Could you check a few things on this model? Use its own coordinates, in mm. Face numbers are marked on the shaded views. A direction names the side the tool comes from. Coordinates: 2 decimals unless noted, no trailing zeros. Loops run counter-clockwise (first coordinate to the right, second up) from the corner with the lowest first, then second, coordinate; pieces in that order, holes last.
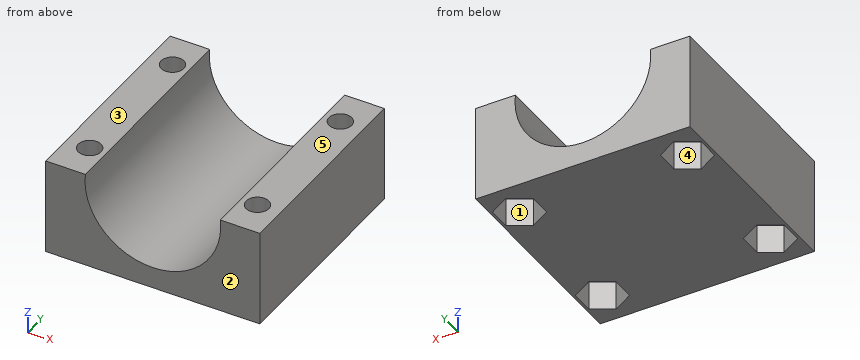
from build123d import *

# Parameters (mm, degrees)
F0_W     = 30
F0_H     = 30
F0_R     = 1.6
F1_DEPTH = 13.5
F2_R     = 9.5
F3_DEPTH = 30.001
F5_DEPTH = 4


with BuildPart() as f1:
    # F0 (on Top) → F1 (new body)
    with BuildSketch(Plane.XY):
        Rectangle(F0_W, F0_H)
        with Locations((-11.75, -10)):
            Circle(F0_R, mode=Mode.SUBTRACT)
        with Locations((11.75, -10)):
            Circle(F0_R, mode=Mode.SUBTRACT)
        with Locations((-11.75, 10)):
            Circle(F0_R, mode=Mode.SUBTRACT)
        with Locations((11.75, 10)):
            Circle(F0_R, mode=Mode.SUBTRACT)
    extrude(amount=F1_DEPTH)

    # F2 (on face) → F3 (cut, through all)
    with BuildSketch(Plane.XZ.offset(15)):
        with Locations((0, 12.5)):
            Circle(F2_R)
    extrude(amount=-F3_DEPTH, mode=Mode.SUBTRACT)

    # F4 (on face) → F5 (cut)
    with BuildSketch(Plane(origin=(0, 0, 0), x_dir=(1, 0, 0), z_dir=(0, 0, -1))):
        Polygon((-8.9, 8.354552), (-8.9, 11.645448), (-11.75, 13.290897), (-14.6, 11.645448), (-14.6, 8.354552), (-11.75, 6.709103), align=None)
        Polygon((14.6, 11.645448), (11.75, 13.290897), (8.9, 11.645448), (8.9, 8.354552), (11.75, 6.709103), (14.6, 8.354552), align=None)
        Polygon((14.6, -11.645448), (14.6, -8.354552), (11.75, -6.709103), (8.9, -8.354552), (8.9, -11.645448), (11.75, -13.290897), align=None)
        Polygon((-11.75, -13.290897), (-8.9, -11.645448), (-8.9, -8.354552), (-11.75, -6.709103), (-14.6, -8.354552), (-14.6, -11.645448), align=None)
    extrude(amount=-F5_DEPTH, mode=Mode.SUBTRACT)


solid = f1.part
1) Imagine slicing it at B-B on y = 10. List the corners of the cut face in (x, z) for me.
2) Imagine slicing it at A-A on z = 12.5. List the corners of the cut face in (x, y) for me.
3) We'd pull the mould along Y, two halves only. Please class the marked faces 1, 2 and 3: released by +Y, released by -Y, zero draft, split by the parting line, or undercut.
4) Will these pins go through, and if not, where does the flat tip stop? pin 1 (1.7 mm diameter, centred on x = -12, y = 10.5, fed in from -Z); pin 2 (5 mm diameter, centred on x = 11.75, y = 10, fed in from -Z).
5) Imagine slicing it at D-D on z = 6.5. List the corners of the cut face in (x, y) for me.
6) If I drill on L1, parallel to Y at x = -11.75, z = 6; L2, parallel to X at y = 6, z = 12.5; L3, parallel to X at y = 10, z = 9, over which ranges is the centre line in solid material (lowest first)?
7) For the marked faces 4 and 5, which set-ups out of +Z, -Z, +X, -X, +Y, -Y let a thin tool reach every point of the face, with its end or its side?
8) Imagine slicing it at C-C on y = 3.5. List the corners of the cut face in (x, z) for me.
Solved:
1. outline: (-15, 0) - (-14.6, 0) - (-14.6, 4) - (-13.35, 4) - (-13.35, 13.5) - (-15, 13.5) - close; (-10.15, 4) - (-8.9, 4) - (-8.9, 0) - (8.9, 0) - (8.9, 4) - (10.15, 4) - (10.15, 13.5) - (9.45, 13.5) arc R9.5 cw (long way) to (-9.45, 13.5) - (-10.15, 13.5) - close; (13.35, 4) - (14.6, 4) - (14.6, 0) - (15, 0) - (15, 13.5) - (13.35, 13.5) - close
2. outline: (-15, -15) - (-9.5, -15) - (-9.5, 15) - (-15, 15) - close; (9.5, -15) - (15, -15) - (15, 15) - (9.5, 15) - close; hole circle Ø3.2 at (-11.75, -10); hole circle Ø3.2 at (-11.75, 10); hole circle Ø3.2 at (11.75, -10); hole circle Ø3.2 at (11.75, 10)
3. face 1: undercut
3. face 2: released by -Y
3. face 3: zero draft
4. pin 1: passes through
4. pin 2: stops at z = 4
5. outline: (-15, -15) - (-7.37, -15) - (-7.37, 15) - (-15, 15) - close; (7.37, -15) - (15, -15) - (15, 15) - (7.37, 15) - close; hole circle Ø3.2 at (-11.75, -10); hole circle Ø3.2 at (-11.75, 10); hole circle Ø3.2 at (11.75, -10); hole circle Ø3.2 at (11.75, 10)
6. L1: y = -15 to -11.6, -8.4 to 8.4, 11.6 to 15
6. L2: x = -15 to -9.5, 9.5 to 15
6. L3: x = -15 to -13.35, -10.15 to -8.83, 8.83 to 10.15, 13.35 to 15
7. face 4: -Z
7. face 5: +Z, +X, -X, +Y, -Y
8. outline: (-15, 0) - (15, 0) - (15, 13.5) - (9.45, 13.5) arc R9.5 cw (long way) to (-9.45, 13.5) - (-15, 13.5) - close
